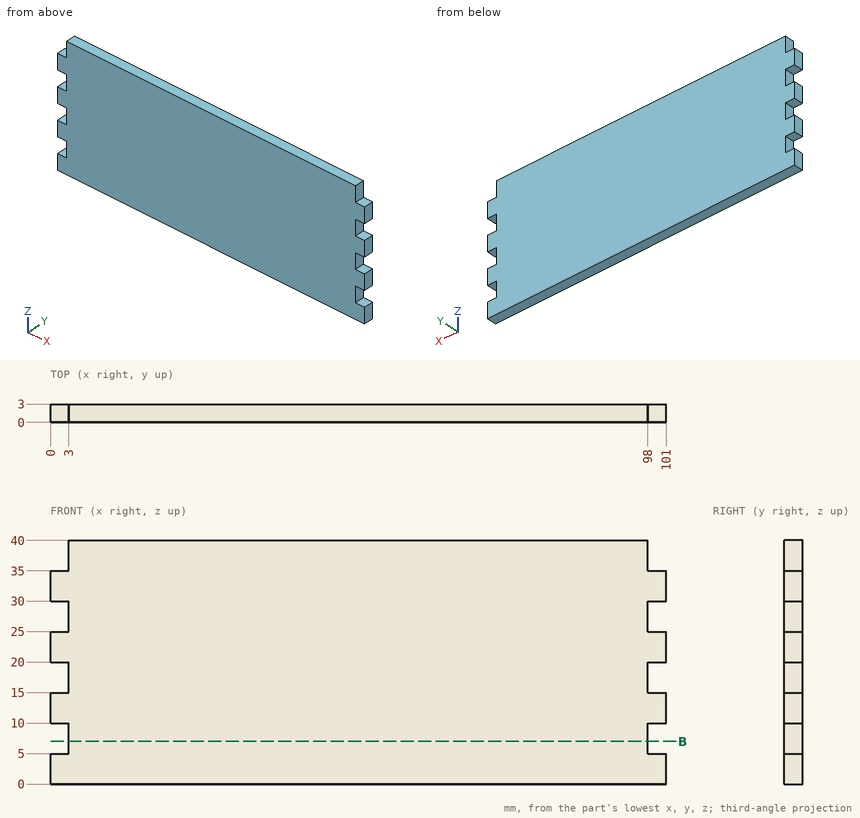
Answer from the drawing. Dimensions are ordinates in mm from the lowest x, y and z of the part. Give positions to 0.01 mm unless a question says otherwise; leave off trailing zeros. Write each loop counter-clockwise with the first axis right and the second up, starting at its lowest first coordinate (ties: lowest second). Pieces come first, ordered by that corner, then holes. Notation, with made-up numbers: (-17, 45.25) - (5, 45.25) arc R20 ccw to (5, 84.25) - close; hole circle Ø8 at (-33.75, -28). An arc over 180 degrees is marked (long way). One line per item, written item: value. Start each with the question number.
1. Given pin 1 (1.5 mm diameter, centred on y = 2.5, z = 26.5, fed in from +X); pin 2 (1.5 mm diameter, centred on x = 99, y = 1.5, fed in from -Z); pin 3 (0.9 mm diameter, centred on y = 2, z = 38.5, fed in from -X); pin 4 (1.5 mm diameter, centred on x = 100, y = 1, fed in from +Z), each flat-ended and moving along its own axis, determine where each tip first touches the part or whether it passes through.
2. Find section B-B (z = 7). Write down the section's boundary in (x, y).
3. Consider probe 1 along X at (y, z) = (2.4, 27). Determine where the line is inside the solid, lowest interval first.
Geometry results:
1. pin 1: x = 98
1. pin 2: z = 0
1. pin 3: x = 3
1. pin 4: z = 35
2. outline: (3, 0) - (98, 0) - (98, 3) - (3, 3) - close
3. probe 1: 3 to 98
